Part model, mm, in its own coordinate system. Round coordinates to 2 decimals unless told otherwise and drop trailing zeros. Write each loop counter-clockwise with the first axis right and the second up, starting at its lowest first coordinate (ties: lowest second). Pieces come first, ordered by that corner, then holes. Notation, with made-up numbers: (80.5, 11) -> (124.5, 11) arc R20 cw to (124.5, 35) -> close; hole circle Ø4 at (70, -18.75). An arc over 180 degrees is marked (long way). Return JSON: item names as keys, results as strings. Group by question number.
(1) Drop flat-ended pins along their axis: pin 1 Ø2 at (x, y) = (10.5, 1) entering from +Z; pin 2 Ø5 at (x, y) = (-24, -4.5) entering from -Z. Give the stop position or say it passes through.
(2) Saw through at A-A (y = -3.5). List the corners of the cut face in (x, z).
(3) Drill centre lines: L1, parallel to Y at x = 31, z = 28; L2, parallel to X at y = -5, z = 45; L3, parallel to Z at x = 23, y = 5. Where is each one in solid material? Low to high. Write a range as from..to.
from build123d import *

# Parameters (mm, degrees)
SKETCH2_W           = 76.2
SKETCH2_H           = 76.2
BOSS_EXTRUDE1_DEPTH = 50.8
SKETCH3_R           = 7.62


with BuildPart() as part:
    # Sketch2 → Boss-Extrude1 (new body)
    with BuildSketch(Plane.XY):
        Rectangle(SKETCH2_W, SKETCH2_H)
    extrude(amount=BOSS_EXTRUDE1_DEPTH)

    # Sketch3 → Cut-Revolve1 (revolve, cut)
    with BuildSketch(Plane.XY.offset(50.8), mode=Mode.PRIVATE) as cut_revolve1_sk:
        with Locations((12.7, 0)):
            Circle(SKETCH3_R)
    revolve(cut_revolve1_sk.sketch.rotate(Axis((38.1, 38.1, 50.8), (0, 1, 0)), 315), axis=Axis((38.1, 38.1, 50.8), (0, 1, 0)), mode=Mode.SUBTRACT)


solid = part.part
Computed values:
{
 "1": {"pin 1": "z = 34.45", "pin 2": "z = 0"},
 "2": {"outline": "(-38.1, 0) -> (38.1, 0) -> (38.1, 18.63) arc R32.17 cw to (5.93, 50.8) -> (-38.1, 50.8) -> close; (19.47, 50.8) arc R18.63 ccw to (38.1, 32.17) -> (38.1, 50.8) -> close"},
 "3": {"L1": "-38.1..-7.47, 7.47..38.1", "L2": "-38.1..7.49, 19.33..38.1", "L3": "0..23.55, 38.23..50.8"}
}
